Build history of the part. All positions in model axes, mm. Face numbers are marked on the shaded views. Round coordinates to 2 decimals unless told otherwise and drop trailing zeros. Write each loop counter-clockwise with the first axis right and the second up, starting at its lowest first coordinate (ties: lowest second). Pieces come first, ordered by that corner, then holes.
Item 1: Band-saw the part on C-C, the plane z = 2.5. Write the cut outline in (x, y).
Item 2: Mould opens along Y. For the marked faces 1, 2 and 3 say: +Y half, -Y half, draft (parallel to the pull), parting line (faces both ways), or undercut.
Item 3: Band-saw the part on B-B, the plane y = 8.5. Write the cut outline in (x, z), then the cut area to 3 significant figures.
Item 4: Drop flat-ended pins along their axis: pin 1 Ø1.5 at (x, y) = (2, 3) entering from +Z; pin 2 Ø1 at (x, z) = (-1.5, 1) entering from +Y; pin 3 Ø4 at (x, y) = (-2.5, 10) entering from -Z; pin 4 Ø2 at (y, z) = (6.5, 0) entering from +X. Give the stop position or say it passes through.
Item 5: Wall check: probe 1 along X at (y, z) = (0, 0.5); probe 2 along Z at (x, y) = (-2.75, 6.5). Give the ranges that are in metal, low to high.
Item 6: Band-saw the part on D-D, the plane y = -3. Write the cut outline in (x, z).
Item 7: Band-saw the part on A-A, the plane x = 0. Write the cut outline in (y, z), then the cut area to 3 significant figures.
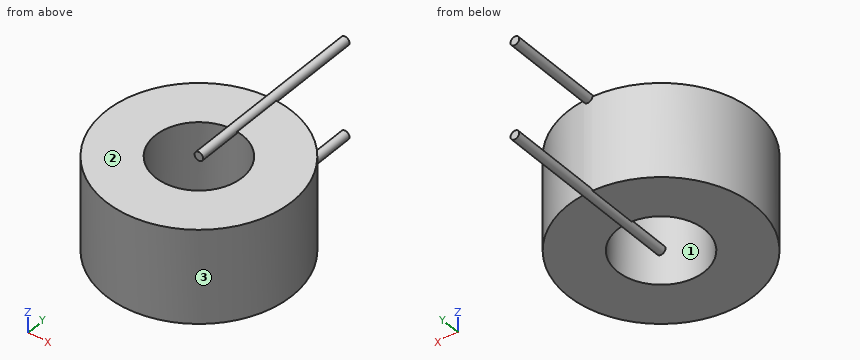
```python
from build123d import *

# Parameters (mm, degrees)
EXTRUDE_1_DEPTH      = 3.8
EXTRUDE_1_DEPTH_BACK = 3.8
SKETCH_1_R           = 7.5
SKETCH_1_R_2         = 3.5
SKETCH_3_R           = 0.35
EXTRUDE_2_DEPTH      = 15


with BuildPart() as part:
    # Sketch 1 → Extrude 1 (new, two sides: drawn at the far end of the back side and taken through both)
    with BuildSketch(Plane.XY.offset(-EXTRUDE_1_DEPTH_BACK)):
        Circle(SKETCH_1_R)
        Circle(SKETCH_1_R_2, mode=Mode.SUBTRACT)
    extrude(amount=EXTRUDE_1_DEPTH + EXTRUDE_1_DEPTH_BACK)

    # Sketch 3 → Extrude 2 (add)
    with BuildSketch(Plane(origin=(0, 0, 0), x_dir=(1, 0, 0), z_dir=(0, 1, 0))):
        with Locations(Location((0, 3.8, 0), (0, 0, 270))):
            Circle(SKETCH_3_R)
        with Locations(Location((0, -3.8, 0), (0, 0, 90))):
            Circle(SKETCH_3_R)
    extrude(amount=EXTRUDE_2_DEPTH)


solid = part.part
```
Results:
1. outline: circle Ø15 at (0, 0); hole circle Ø7 at (0, 0)
2. face 1: undercut
2. face 2: draft
2. face 3: parting line
3. outline: circle Ø0.7 at (0, -3.8); circle Ø0.7 at (0, 3.8)
3. area: 0.770 mm2
4. pin 1: stops at z = 3.8
4. pin 2: stops at y = 7.43
4. pin 3: passes through
4. pin 4: stops at x = 5.1
5. probe 1: x = -7.5 to -3.5, 3.5 to 7.5
5. probe 2: z = -3.8 to 3.8
6. outline: (-6.87, -3.8) - (-1.8, -3.8) - (-1.8, 3.8) - (-6.87, 3.8) - close; (1.8, -3.8) - (6.87, -3.8) - (6.87, 3.8) - (1.8, 3.8) - close
7. outline: (-7.5, -3.8) - (-3.5, -3.8) - (-3.5, 3.8) - (-7.5, 3.8) - close; (0, -4.15) - (15, -4.15) - (15, -3.45) - (7.5, -3.45) - (7.5, 3.45) - (15, 3.45) - (15, 4.15) - (0, 4.15) - (0, 3.45) - (3.5, 3.45) - (3.5, -3.45) - (0, -3.45) - close
7. area: 79.0 mm2
